from build123d import *

# Parameters (mm, degrees)
PAD_DEPTH       = 69
POCKET_DEPTH    = 57
POCKET001_DEPTH = 10
PAD001_DEPTH    = 5
POCKET002_DEPTH = 24.001
POCKET003_DEPTH = 24.001
SKETCH006_R     = 12
PAD002_DEPTH    = 10
SKETCH007_R     = 9.1
PAD003_DEPTH    = 4.3


with BuildPart() as part:
    # Sketch → Pad (new body)
    with BuildSketch(Plane.XZ):
        with BuildLine():
            Line((-24, -12.5), (-24, 8.5))
            ThreePointArc((-20, 12.5), (-22.828427, 11.328427), (-24, 8.5))
            Line((-20, 12.5), (20, 12.5))
            ThreePointArc((24, 8.5), (22.828427, 11.328427), (20, 12.5))
            Line((24, 8.5), (24, -12.5))
            ThreePointArc((-24, -12.5), (0, -16.5), (24, -12.5))
        make_face()
    extrude(amount=-PAD_DEPTH)

    # Sketch001 → Pocket (cut)
    with BuildSketch(Plane.XZ.offset(-10)):
        with BuildLine():
            Line((-12, -5.5), (-12, 12.5))
            Line((-12, 12.5), (12, 12.5))
            Line((12, 12.5), (12, -5.5))
            ThreePointArc((8, -9.5), (10.828427, -8.328427), (12, -5.5))
            Line((8, -9.5), (-8, -9.5))
            ThreePointArc((-12, -5.5), (-10.828427, -8.328427), (-8, -9.5))
        make_face()
    extrude(amount=-POCKET_DEPTH, mode=Mode.SUBTRACT)

    # Sketch002 → Pocket001 (cut)
    with BuildSketch(Plane.XZ):
        with BuildLine():
            ThreePointArc((-3.25, 3.112475), (0, -4.5), (3.25, 3.112475))
            Line((8.66989, 12.5), (3.25, 3.112475))
            Line((-8.66989, 12.5), (8.66989, 12.5))
            Line((-3.25, 3.112475), (-8.66989, 12.5))
        make_face()
    extrude(amount=-POCKET001_DEPTH, mode=Mode.SUBTRACT)

    # Sketch003 → Pad001 (join)
    with BuildSketch(Plane.XZ):
        with BuildLine():
            ThreePointArc((-3.25, 3.112475), (0, -4.5), (3.25, 3.112475))
            Line((7.559237, 10.576292), (3.25, 3.112475))
            ThreePointArc((-7.559237, 10.576292), (0, -13), (7.559237, 10.576292))
            Line((-7.559237, 10.576292), (-3.25, 3.112475))
        make_face()
    extrude(amount=PAD001_DEPTH)

    # Sketch004 → Pocket002 (cut, through all)
    with BuildSketch(Plane.YZ):
        Polygon((69, 12.5), (69, 0), (46.356987, 2.26935), (37, 12.5), align=None)
    extrude(amount=POCKET002_DEPTH, mode=Mode.SUBTRACT)

    # Sketch005 → Pocket003 (cut, through all)
    with BuildSketch(Plane.YZ):
        Polygon((47, 12.5), (57.366132, 1.165981), (69, 0), (69, 12.5), align=None)
    extrude(amount=-POCKET003_DEPTH, mode=Mode.SUBTRACT)

    # Sketch006 → Pad002 (join)
    with BuildSketch(Plane.YZ.offset(-28)):
        with Locations((36, 0)):
            Circle(SKETCH006_R)
    extrude(amount=PAD002_DEPTH)

    # Sketch007 → Pad003 (join)
    with BuildSketch(Plane.YZ.offset(-28)):
        with Locations((36, 0)):
            Circle(SKETCH007_R)
    extrude(amount=-PAD003_DEPTH)


solid = part.part
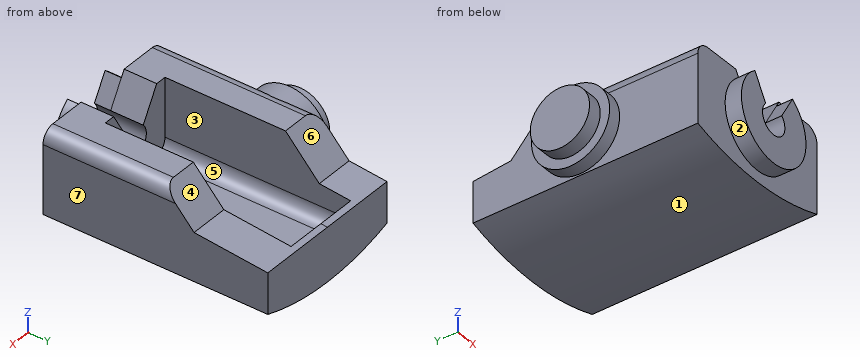
Can you work these out from the model? Positions are in its coordinate system, mm. Face numbers are marked on the shaded views. A direction names the side the tool comes from. Round coordinates to 2 decimals unless told otherwise and drop trailing zeros. Loops run counter-clockwise (first coordinate to the right, second up) from the corner with the lowest first, then second, coordinate; pieces in that order, holes last. Notation, with made-up numbers: (-35.5, -38.75) - (-15.5, -38.75) arc R18 cw to (-15.5, -11.75) - close; hole circle Ø5 at (-19.5, 17.25). An arc over 180 degrees is marked (long way). Write item = value, one per line. Start each with the question number.
(1) If I drill on probe 1 along X at (y, z) = (5.5, 0); probe 2 along X at (y, z) = (-0.25, 0); probe 3 along Y at (x, z) = (-4, -2.25), over which ranges is the centre line in solid material (lowest first)? Write a range as [from, to].
(2) If we section it at C-C (x = -16): Please give me the cut outline in (y, z), and give its area (3 significant figures).
(3) If we section it at A-A (y = 36): Please give me the cut outline in (x, z), and give its area (3 significant figures).
(4) If we mould it in two halves opening along X, with no side actions, what happens to the marked faces 5, 6 and 7? For each: released by +X, released by -X, zero draft, split by the parting line, or undercut.
(5) If we section it at D-D (y = 11): Please give me the cut outline in (x, z).
(6) If we section it at B-B (z = 7.25): Please give me the cut outline in (x, y), and give its area (3 significant figures).
(7) For P1, Ø12, axis at y = 8, z = -5.5, coming from the -X side; P2, Ø1, axis at x = -9.5, y = 22.5, coming from the -Z side; P3, Ø13, axis at x = -0.5, y = 25.5, coming from the +Z side, each with a flat end and sliding along its axis, tell me the tip position at first contact or that it passes through.
(8) For the marked faces 1, 2, 3 and 4, which set-ups out of +Z, -Z, +X, -X, +Y, -Y let a thin tool reach every point of the face, with its end or its side?
Ans:
q1.probe_1 = [-24, -4.5], [4.5, 24]
q1.probe_2 = [-13, -4.5], [4.5, 13]
q1.probe_3 = [-5, 10], [67, 69]
q2.outline = (0, -14.75) - (69, -14.75) - (69, 0) - (57.37, 1.17) - (47, 12.5) - (0, 12.5) - close
q2.area = 1,680 mm²
q3.outline = (-32.3, -9.1) - (-28, -9.1) - (-28, -12) - (-24, -12) - (-24, -12.5) arc R74 ccw to (24, -12.5) - (24, 8.5) arc R4 ccw to (20, 12.5) - (12, 12.5) - (12, -5.5) arc R4 cw to (8, -9.5) - (-8, -9.5) arc R4 cw to (-12, -5.5) - (-12, 12.5) - (-20, 12.5) arc R4 ccw to (-21.94, 12) - (-28, 12) - (-28, 9.1) - (-32.3, 9.1) - close
q3.area = 977 mm²
q4.face_5 = undercut
q4.face_6 = zero draft
q4.face_7 = released by +X
q5.outline = (-24, -12.5) arc R74 ccw to (24, -12.5) - (24, 8.5) arc R4 ccw to (20, 12.5) - (12, 12.5) - (12, -5.5) arc R4 cw to (8, -9.5) - (-8, -9.5) arc R4 cw to (-12, -5.5) - (-12, 12.5) - (-20, 12.5) arc R4 ccw to (-24, 8.5) - close
q6.outline = (-32.3, 30.5) - (-28, 30.5) - (-28, 26.44) - (-24, 26.44) - (-24, 0) - (-10.79, 0) - (-10.79, -5) - (-5.64, -5) - (-5.64, 10) - (-12, 10) - (-12, 51.8) - (-24, 51.8) - (-24, 45.56) - (-28, 45.56) - (-28, 41.5) - (-32.3, 41.5) - close; (5.64, -5) - (10.79, -5) - (10.79, 0) - (24, 0) - (24, 41.8) - (12, 41.8) - (12, 10) - (5.64, 10) - close
q6.area = 1,430 mm²
q7.P1 = -24
q7.P2 = -15.95
q7.P3 = -9.5
q8.face_1 = -Z, +Y, -Y
q8.face_2 = -Y
q8.face_3 = +Z
q8.face_4 = +Z, +X, +Y
